Work out the finished part from the listing and answer in its coordinate system (mm). A direction names the side the tool comes from. Give positions to 0.01 mm unless a question says otherwise; leave off trailing zeros. Order: outer loops, then holes, each group sorted by start corner. A loop starts at its lowest first (then second) coordinate and runs counter-clockwise, first axis right, second up. Notation, with made-up numbers: (-21.5, 78) - (25.5, 78) arc R24 cw to (25.5, 90) - close; hole circle Ø7 at (79, -25.75). An arc over 180 degrees is marked (long way). Put each result on its own line as item: value.
```python
from build123d import *

# Parameters (mm, degrees)
F0_W     = 76.2
F0_H     = 25.4
F1_DEPTH = 10.16
F2_R     = 6.35
F3_DEPTH = 3.81


# Not quite as in the source:
# - a pattern or mirror of a feature is missing from the dataset's text; its kind, count and spacing are read off the source's solid


with BuildPart() as f1:
    # F0 (on Top) → F1 (new body)
    with BuildSketch(Plane.XY):
        Rectangle(F0_W, F0_H)
    extrude(amount=F1_DEPTH)

    # F2 (on face) → F3 (cut)
    with BuildSketch(Plane(origin=(0, 0, 0), x_dir=(1, 0, 0), z_dir=(0, 0, -1))):
        with Locations((-23.495, 0)):
            Circle(F2_R)
        with Locations((-3.175, 0)):
            Circle(F2_R)
        with Locations((17.145, 0)):
            Circle(F2_R)
    extrude(amount=-F3_DEPTH, mode=Mode.SUBTRACT)

    # F5 (on offset) → F6 (revolve, cut)
    with BuildSketch(Plane.XZ.offset(3.81)):
        Polygon((-26.035, 3.81), (-23.495, 3.81), (-23.495, 10.4205608368), (-24.257, 10.4205608368), (-24.257, 4.4571390765), align=None)
    f6 = revolve(axis=Axis((-23.495, -3.81, 7.1152804184), (0, 0, -1)), mode=Mode.SUBTRACT)

    # F6_copies: F6 across plane
    add(f6.mirror(Plane.ZX), mode=Mode.SUBTRACT)

    # F7 (on offset) → F8 (revolve, cut)
    with BuildSketch(Plane.XZ.offset(3.81)):
        Polygon((-5.715, 3.81), (-3.175, 3.81), (-3.175, 10.4205607442), (-3.937, 10.4205607442), (-3.937, 4.4571389839), align=None)
    f8 = revolve(axis=Axis((-3.175, -3.81, 10.0472030926), (0, 0, 1)), mode=Mode.SUBTRACT)

    # F8_copies: F8 across plane
    add(f8.mirror(Plane.ZX), mode=Mode.SUBTRACT)

    # F9 (on offset) → F10 (revolve, cut)
    with BuildSketch(Plane.XZ.offset(3.81)):
        Polygon((14.605, 3.81), (17.145, 3.81), (17.145, 10.4205608368), (16.383, 10.4205608368), (16.383, 4.4571390765), align=None)
    f10 = revolve(axis=Axis((17.145, -3.81, 8.0366932552), (0, 0, 1)), mode=Mode.SUBTRACT)

    # F10_copies: F10 across plane
    add(f10.mirror(Plane.ZX), mode=Mode.SUBTRACT)


solid = f1.part
```
(1) Section A-A, the plane z = 1.75 is taken. Write down the section's boundary in (x, y) (3 decimals), then the cut area to 3 significant figures.
Geometry check:
outline: (-38.1, -12.7) - (38.1, -12.7) - (38.1, 12.7) - (-38.1, 12.7) - close; hole circle Ø12.7 at (-23.495, 0); hole circle Ø12.7 at (-3.175, 0); hole circle Ø12.7 at (17.145, 0)
area: 1,560 mm²
(2) Section B-B, the plane y = 0 is taken. Write down the section's boundary in (x, z) (3 decimals).
Geometry check:
outline: (-38.1, 0) - (-29.845, 0) - (-29.845, 3.81) - (-17.145, 3.81) - (-17.145, 0) - (-9.525, 0) - (-9.525, 3.81) - (3.175, 3.81) - (3.175, 0) - (10.795, 0) - (10.795, 3.81) - (23.495, 3.81) - (23.495, 0) - (38.1, 0) - (38.1, 10.16) - (-38.1, 10.16) - close
(3) Section C-C, the plane y = 3.81 is taken. Count the separate pieces of the cut face and the enclosed holes in it, then the cut area to 3 significant figures.
Geometry check:
separate pieces: 4
enclosed holes: 0
area: 626 mm²
(4) Determine the mould class of faces 3 (the face through (-1, -12.7, 5)), 4 (the face through (-3.527, 3.134, 7.269)), 5 (the face through (-1, 12.7, 5)) for opening direction Y: pulls with the +Y half, pulls with the -Y half, needs draft (parallel to the pull), parting line crosses it, or undercut.
Geometry check:
face 3: pulls with the -Y half
face 4: undercut
face 5: pulls with the +Y half
(5) A tool of negligible diameter and unlimited length cuts with its end or side. For faces 1 (the face through (-3, 0, 3.81)), 2 (the face through (-38.1, 0, 5)), from which of +Z, -Z, +X, -X, +Y, -Y can it reach the whole face along a straight path? Write none if from no direction.
Geometry check:
face 1: -Z
face 2: +Z, -Z, -X, +Y, -Y
(6) Given pin 1 (6.5 mm diameter, centred on x = 15, y = 0, fed in from -Z); pin 2 (1.8 mm diameter, centred on x = -23.495, y = 3.81, fed in from -Z), each flat-ended and moving along its own axis, determine where each tip first touches the part or whether it passes through.
Geometry check:
pin 1: stops at z = 3.81
pin 2: stops at z = 4.41
(7) Straight lines are drawn through the part: line 1 (X direction, y = 0, z = 1.1) (3 decimals); line 2 (Y direction, x = -23.5, z = 7); line 3 (X direction, y = 0.75, z = 1.75). For each, find the intervals that lie inside material, in ascending order.
Geometry check:
line 1: x = -38.1 to -29.845, -17.145 to -9.525, 3.175 to 10.795, 23.495 to 38.1
line 2: y = -12.7 to -4.57, -3.05 to 3.05, 4.57 to 12.7
line 3: x = -38.1 to -29.8, -17.19 to -9.48, 3.13 to 10.84, 23.45 to 38.1
